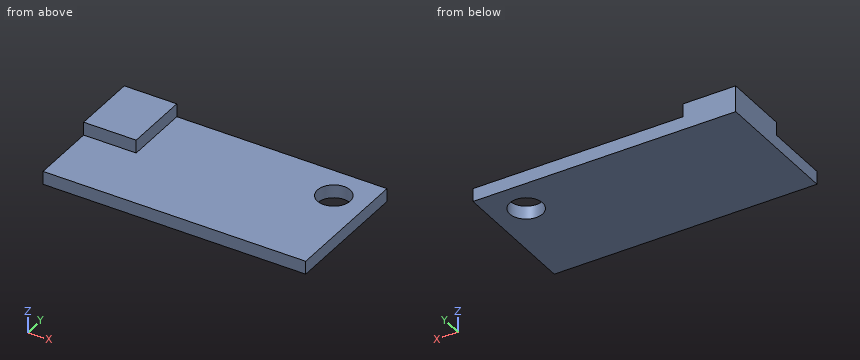
from build123d import *

# Parameters (mm, degrees)
CROQUIS2_W              = 200
CROQUIS2_H              = 100
CROQUIS2_R              = 12.5
SALIENTE_EXTRUIR5_DEPTH = 10
CROQUIS11_W             = 40
CROQUIS11_H             = 50
SALIENTE_EXTRUIR6_DEPTH = 10


with BuildPart() as part:
    # Croquis2 → Saliente-Extruir5 (new body)
    with BuildSketch(Plane.XY):
        with Locations((100, 50)):
            Rectangle(CROQUIS2_W, CROQUIS2_H)
        with Locations((175, 75)):
            Circle(CROQUIS2_R, mode=Mode.SUBTRACT)
    extrude(amount=SALIENTE_EXTRUIR5_DEPTH)

    # Croquis11 → Saliente-Extruir6 (add)
    with BuildSketch(Plane.XY.offset(10)):
        with Locations((20, 75)):
            Rectangle(CROQUIS11_W, CROQUIS11_H)
    extrude(amount=SALIENTE_EXTRUIR6_DEPTH)


solid = part.part
Source: CAD feature listing. Evaluate the final solid. Frame: model axes, mm. Give positions to 0.01 mm unless a question says otherwise; leave off trailing zeros. Write each loop counter-clockwise with the first axis right and the second up, starting at its lowest first coordinate (ties: lowest second). Pieces come first, ordered by that corner, then holes. Notation, with made-up numbers: M 78.5,66 L 108.5,66 A7 cw 108.5,70 Z; hole C 59.5,-1.75 d3. An arc over 180 degrees is marked long. Return JSON: item names as keys, results as strings. Group by question number.
1) Cut plane D-D, the plane x = 144. Output: boundary loops of the cut face in (y, z).
2) Cut plane C-C, the plane z = 6.5. Output: boundary loops of the cut face in (x, y), then the cut area to 3 significant figures.
3) Cut plane B-B, the plane y = 75. Output: boundary loops of the cut face in (x, z).
4) Cut plane A-A, the plane x = 175. Output: boundary loops of the cut face in (y, z), then the cut area to 3 significant figures.
5) First-contact query: pin 1 Ø11 at (y, z) = (74.5, 16.5) entering from +X; pin 2 Ø1 at (x, y) = (84.5, 27) entering from +Z. Flat tips, straight axial feed; report the tip coordinate or a pass-through.
6) Ray query, L1, parallel to Y at x = 175, z = 6; L2, parallel to X at y = 74, z = 15; L3, parallel to Z at x = 14, y = 37. Return the intervals inside material, ascending.
Data:
{
 "1": {"outline": "M 0,0 L 100,0 L 100,10 L 0,10 Z"},
 "2": {"outline": "M 0,0 L 200,0 L 200,100 L 0,100 Z; hole C 175,75 d25", "area": "19,500 mm²"},
 "3": {"outline": "M 0,0 L 162.5,0 L 162.5,10 L 40,10 L 40,20 L 0,20 Z; M 187.5,0 L 200,0 L 200,10 L 187.5,10 Z"},
 "4": {"outline": "M 0,0 L 62.5,0 L 62.5,10 L 0,10 Z; M 87.5,0 L 100,0 L 100,10 L 87.5,10 Z", "area": "750 mm²"},
 "5": {"pin 1": "stops at x = 40", "pin 2": "stops at z = 10"},
 "6": {"L1": "y = 0 to 62.5, 87.5 to 100", "L2": "x = 0 to 40", "L3": "z = 0 to 10"}
}
